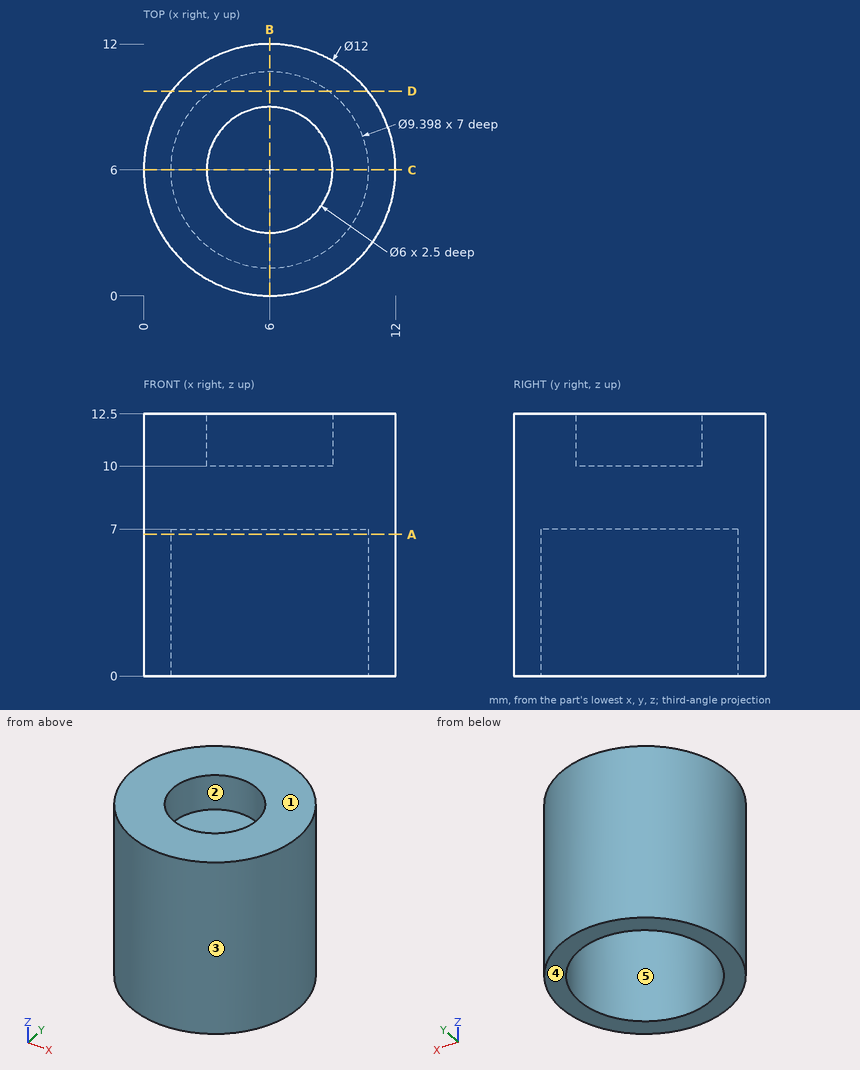
Geometry: see drawing. Coordinates: mm, zero at the bounding-box minimum. A direction names the side the tool comes from. Round coordinates to 2 decimals unless told otherwise and drop trailing zeros. Write each loop counter-clockwise with the first axis right and the second up, starting at its lowest first coordinate (ties: lowest second). Pieces come first, ordered by that corner, then holes.
1) Ray query, L1, parallel to Y at x = 6, z = 2.5; L2, parallel to Y at x = 6, z = 11.7; L3, parallel to Z at x = 10, y = 5.75. Return the intervals inside material, ascending.
2) Draft query along X for the marked faces 3, 4 and 5. Return one class per face: pulls with the +X half, pulls with the -X half, needs draft (parallel to the pull), parting line crosses it, or undercut.
3) Cut plane B-B (x = 6). Return the cut outline in (y, z), then the cut area to 3 significant figures.
4) Cut plane D-D (y = 9.75). Return the cut outline in (x, z), then the cut area to 3 significant figures.
5) Reachability of the marked faces 1 and 2 from +Z, -Z, +X, -X, +Y, -Y: full face, straight path, thin tool, end or side. Return the list, or none.
6) Contact query for flat-ended pins moving along their axis: P1, Ø6, axis at x = 2, z = 6, coming from the -Y side; P2, Ø4, axis at y = 1.5, z = 6, coming from the +X side; P3, Ø3.5, axis at x = 6, y = 6, coming from the -Z side. Output: stop coordinate, or through.
7) Cut plane A-A (z = 6.75). Return the cut outline in (x, y).
Geometry says:
1. L1: y = 0 to 1.3, 10.7 to 12
1. L2: y = 0 to 3, 9 to 12
1. L3: z = 7 to 12.5
2. face 3: parting line crosses it
2. face 4: needs draft
2. face 5: undercut
3. outline: (0, 0) - (1.3, 0) - (1.3, 7) - (10.7, 7) - (10.7, 0) - (12, 0) - (12, 12.5) - (9, 12.5) - (9, 10) - (3, 10) - (3, 12.5) - (0, 12.5) - close
3. area: 69.2 mm2
4. outline: (1.32, 0) - (3.17, 0) - (3.17, 7) - (8.83, 7) - (8.83, 0) - (10.68, 0) - (10.68, 12.5) - (1.32, 12.5) - close
4. area: 77.5 mm2
5. face 1: +Z, +X, -X, +Y, -Y
5. face 2: +Z
6. P1: stops at y = 0.08
6. P2: stops at x = 11.45
6. P3: stops at z = 7
7. outline: circle Ø12 at (6, 6); hole circle Ø9.4 at (6, 6)
